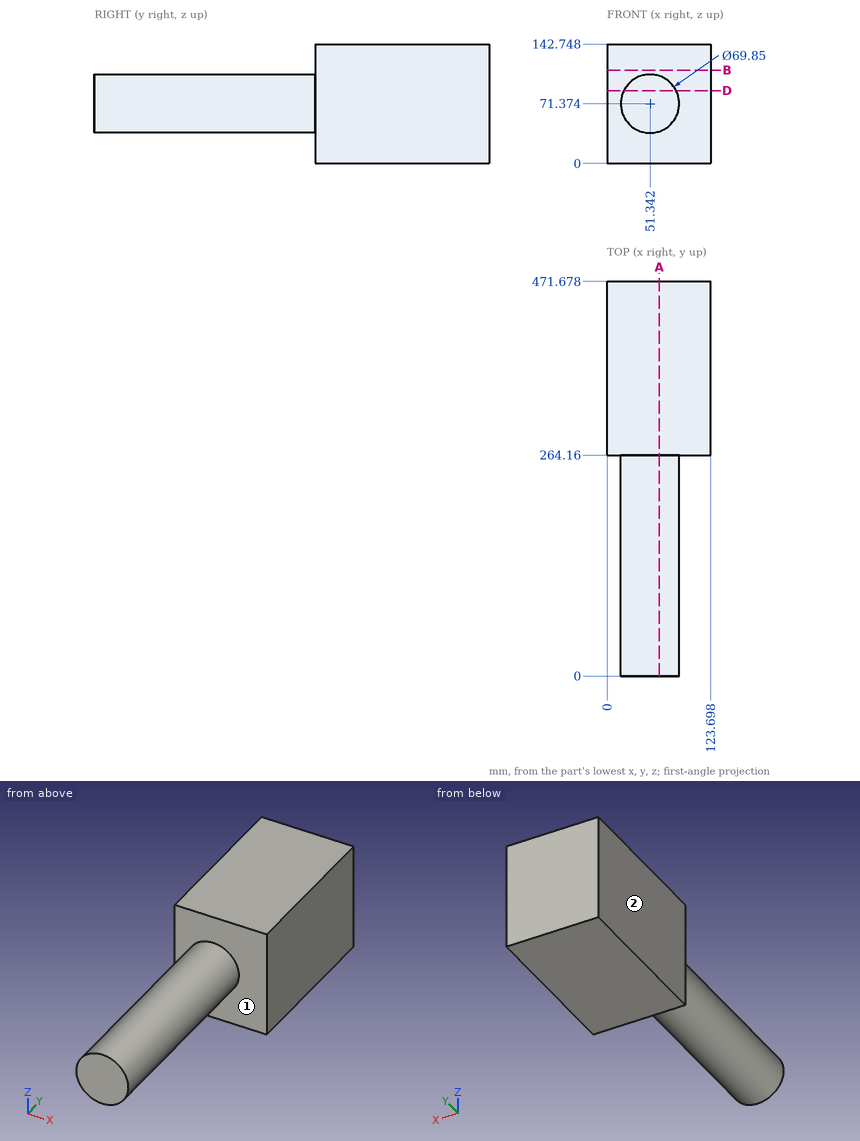
The figure shows three views and two pictorial views of one solid part (mm, origin at its lowest corner). Answer the questions. A direction names the side the tool comes from. Coordinates: 2 decimals unless noted, no trailing zeros. Loops run counter-clockwise (first coordinate to the right, second up) from the corner with the lowest first, then second, coordinate; pieces in that order, holes last. Notation, with made-up numbers: (37.25, 34.5) -> (48.25, 34.5) arc R19 cw to (48.25, 67.5) -> close; hole circle Ø9 at (70.5, 6.25). An arc over 180 degrees is marked (long way). Write item = value, one per line. Start each with the question number.
1) A cutting plane is placed at A-A (x = 62.5). Give the vertices of the cut face in (y, z).
2) Straight lines are drawn through the part: line 1 (Y direction, x = 117, z = 22.5); line 2 (X direction, y = 134.5, z = 73.5); line 3 (X direction, y = 121, z = 101) (1 decimal). For each, find the intervals that lie inside material, in ascending order. Write a range as from..to.
3) A cutting plane is placed at D-D (z = 87). Give the vertices of the cut face in (x, y), then the cut area to 3 significant figures.
4) Given pin 1 Ø3 at (y, z) = (111, 86.5) entering from +X; pin 2 Ø4 at (x, y) = (49.5, 194.5) entering from +Z; pin 3 Ø1 at (y, z) = (176.5, 56.5) entering from -X, each flat-ended and moving along its own axis, determine where each tip first touches the part or whether it passes through.
5) A tool of negligible diameter and unlimited length cuts with its end or side. For the marked faces 1 and 2, from which of +Z, -Z, +X, -X, +Y, -Y can it reach the whole face along a straight path? Write none if from no direction.
6) A cutting plane is placed at B-B (z = 111.5). Give the vertices of the cut face in (x, y).
Responses:
q1.outline = (0, 38.28) -> (264.16, 38.28) -> (264.16, 0) -> (471.68, 0) -> (471.68, 142.75) -> (264.16, 142.75) -> (264.16, 104.47) -> (0, 104.47) -> close
q2.line_1 = 264.16..471.68
q2.line_2 = 16.48..86.2
q2.line_3 = 32.8..69.8
q3.outline = (0, 264.16) -> (20.11, 264.16) -> (20.11, 0) -> (82.58, 0) -> (82.58, 264.16) -> (123.7, 264.16) -> (123.7, 471.68) -> (0, 471.68) -> close
q3.area = 42,200 mm²
q4.pin_1 = 83.5
q4.pin_2 = 106.3
q4.pin_3 = 19.51
q5.face_1 = -Y
q5.face_2 = +Z, -Z, -X, +Y, -Y
q6.outline = (0, 264.16) -> (123.7, 264.16) -> (123.7, 471.68) -> (0, 471.68) -> close
